Read the model definition and answer for the solid it produces. Units are mm, in the model's axes. A direction names the side the tool comes from. Give positions to 0.01 mm unless a question says otherwise; leave off trailing zeros. Order: outer loops, then holes, each group sorted by start corner. A loop starts at its lowest first (then second) coordinate and runs counter-clockwise, first axis right, second up.
```python
from build123d import *

# Parameters (mm, degrees)
PAD044_DEPTH = 6
PAD045_DEPTH = 6
PAD046_DEPTH = 6
PAD047_DEPTH = 6
PAD048_DEPTH = 6
PAD039_DEPTH = 33
FILLET021_R  = 3
FILLET022_R  = 3


with BuildPart() as pad044:
    # Sketch048 → Pad044 (new body)
    with BuildSketch(Plane.XZ.offset(8)):
        Polygon((-14.595035, 49.426792), (-21.11467, 37.733963), (4.396957, 17.395527), (4.396957, 50.985836), align=None)
    extrude(amount=PAD044_DEPTH)


with BuildPart() as pad045:
    # Sketch049 → Pad045 (new body)
    with BuildSketch(Plane.XZ.offset(4)):
        Polygon((-44.716217, 4.039343), (-16.086502, -8.007815), (-47.125652, -16.724289), align=None)
    extrude(amount=PAD045_DEPTH)


with BuildPart() as pad046:
    # Sketch050 → Pad046 (new body)
    with BuildSketch(Plane.XZ.offset(24)):
        Polygon((-44.716217, 4.039343), (-16.086502, -8.007815), (-47.125652, -16.724289), align=None)
    extrude(amount=PAD046_DEPTH)


with BuildPart() as pad047:
    # Sketch051 → Pad047 (new body)
    with BuildSketch(Plane.XZ.offset(14)):
        Polygon((5.367801, 13.680764), (-7.457918, 6.840382), (-11.733156, -9.120509), (13.253242, -11.590648), (11.448138, 11.685653), align=None)
    extrude(amount=PAD047_DEPTH)


with BuildPart() as pad048:
    # Sketch052 → Pad048 (new body)
    with BuildSketch(Plane.XZ.offset(24)):
        Polygon((5.367801, 13.680764), (-7.457918, 6.840382), (-11.733156, -9.120509), (13.253242, -11.590648), (11.448138, 11.685653), align=None)
    extrude(amount=PAD048_DEPTH)


with BuildPart() as cut019:
    # Sketch044 → Pad039 (new body)
    with BuildSketch(Plane(origin=(0, 0, 0), x_dir=(0.848048, 0, 0.529919), z_dir=(0, -1, 0))):
        Polygon((-40.765351, 19.72502), (-40.765351, 12.915253), (-0.082344, -5.035194), (5.261885, -2.605449), (20.317712, 40.085552), (14.098928, 44.660699), align=None)
    extrude(amount=PAD039_DEPTH)

    # Fillet021
    fillet021_edges = [cut019.edges().sort_by_distance(p)[0] for p in [
        (-4.011709, -16.5, 44.761223),
        (-11.709995, -16.5, 45.345714),
    ]]
    fillet(fillet021_edges, radius=FILLET021_R)

    # Fillet022
    fillet022_edges = [cut019.edges().sort_by_distance(p)[0] for p in [
        (5.843009, -16.5, 0.578828),
        (2.598414, -16.5, -4.313722),
        (-41.41502, -16.5, -10.649589),
        (-45.023647, -16.5, -4.874579),
    ]]
    fillet(fillet022_edges, radius=FILLET022_R)

    # Cut011: cut Pad048
    add(pad048.part, mode=Mode.SUBTRACT)

    # Cut012: cut Pad047
    add(pad047.part, mode=Mode.SUBTRACT)

    # Cut013: cut Pad046
    add(pad046.part, mode=Mode.SUBTRACT)

    # Cut014: cut Pad045
    add(pad045.part, mode=Mode.SUBTRACT)

    # Cut019: cut Pad044
    add(pad044.part, mode=Mode.SUBTRACT)


solid = cut019.part
```
1) Consider L1, parallel to Y at x = -8.5, z = 39.5; L2, parallel to X at y = -9, z = 8.5; L3, parallel to X at y = -6.5, z = 16. Determine where each line is inside the solid, lowest interval first.
Final values:
L1: y = -33 to -14, -8 to 0
L2: x = -36.15 to 4.08
L3: x = -31.18 to 2.4
2) The part is cut by section C-C on x = -22.5. Determine the outline of the cut face in (y, z), and give its area (3 significant figures).
Final values:
outline: (-33, -7.93) - (-30, -7.93) - (-30, -5.31) - (-24, -5.31) - (-24, -7.93) - (-10, -7.93) - (-10, -5.31) - (-4, -5.31) - (-4, -7.93) - (0, -7.93) - (0, 29.08) - (-33, 29.08) - close
area: 1,190 mm2
3) The part is cut by section A-A on y = -9. Determine the outline of the cut face in (x, z), and give its area (3 significant figures).
Final values:
outline: (-40.33, 2.2) - (-17.86, -7.26) - (1.27, -4.51) arc R3 ccw to (3.34, -3.19) - (5.14, -0.49) arc R3 ccw to (5.56, 1.83) - (1.59, 19.63) - (-18.27, 35.46) - close
area: 1,190 mm2
4) For a pull along Y with two mould halves and no side action, classify faces 4 (the face through (-14, -33, 15)), 5 (the face through (-44.456, -2.028, -4.906)), 6 (the face through (-34, -30, -5)) as released by +Y, released by -Y, zero draft, split by the parting line, or undercut.
Final values:
face 4: released by -Y
face 5: zero draft
face 6: undercut
5) A tool of negligible diameter and unlimited length cuts with its end or side. For faces 1 (the face through (-3, -24, 1)), 2 (the face through (-8, -8, 35)), 3 (the face through (-34, -24, -5)), from which of +Z, -Z, +X, -X, +Y, -Y can it reach the whole face along a straight path? Write none if from no direction.
Final values:
face 1: -Z, +X
face 2: +Z, +X
face 3: -Z, -X
6) The part is cut by section D-D on z = 21.5. Determine the outline of the cut face in (x, y).
Final values:
outline: (-27.53, -33) - (1.18, -33) - (1.18, -14) - (-0.75, -14) - (-0.75, -8) - (1.18, -8) - (1.18, 0) - (-27.53, 0) - close
7) The part is cut by section B-B on z = 39. Determine the outline of the cut face in (x, y), and give its area (3 significant figures).
Final values:
outline: (-15.92, -33) - (-2.73, -33) - (-2.73, -14) - (-15.92, -14) - close; (-15.92, -8) - (-2.73, -8) - (-2.73, 0) - (-15.92, 0) - close
area: 356 mm2
8) Given pin 1 (4 mm diameter, centred on x = -27.5, z = 26.5, fed in from -Y) (1 decimal); pin 2 (4 mm diameter, centred on y = -17, z = 25, fed in from -X); pin 3 (4 mm diameter, centred on y = -9.5, z = 13.5, fed in from -X); pin 4 (1.5 mm diameter, centred on y = -13, z = 13, fed in from -X), each flat-ended and moving along its own axis, determine where each tip first touches the part or whether it passes through.
Final values:
pin 1: passes through
pin 2: stops at x = -26.53
pin 3: stops at x = -34.16
pin 4: stops at x = -33.66
